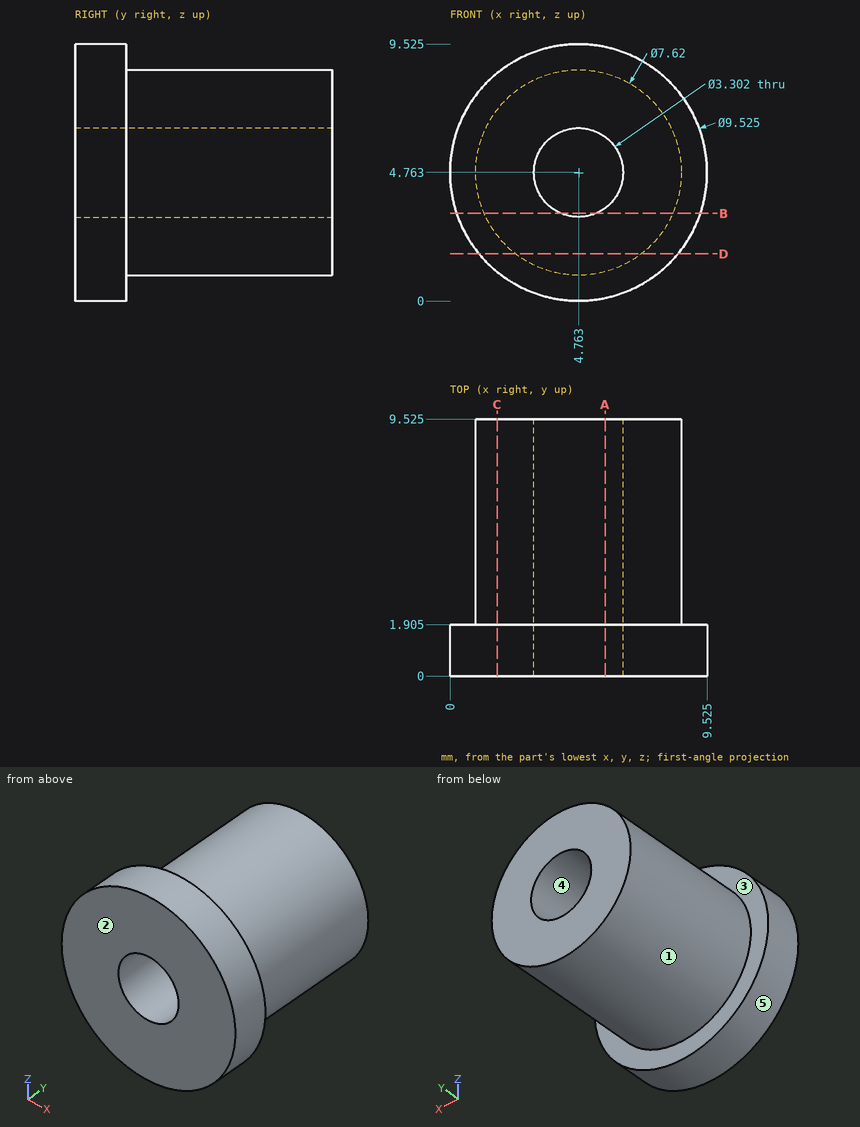
Geometry check sheet. Reference: drawing and pictorial views, mm from the part's lowest x, y, z. A direction names the side the tool comes from. Give positions to 0.01 mm unless a question says otherwise; leave off trailing zeros. Order: outer loops, then holes, each group sorted by start corner. A loop starts at its lowest first (then second) coordinate and runs counter-clockwise, first axis right, second up. Notation, with made-up numbers: M 8,31.5 L 54,31.5 A18 ccw 54,53.5 Z; hole C 40.25,58.5 d9. An arc over 180 degrees is marked long. Use one line per item in the form item = value. Start each with the question number.
Q1. Go/stop test with flat-tipped pins: pin 1 Ø1.5 at (y, z) = (5, 3) entering from -X; pin 2 Ø2 at (x, y) = (2.5, 1.5) entering from +Z (1 decimal); pin 3 Ø2 at (x, z) = (4.76, 4.76) entering from +Y; pin 4 Ø1.5 at (y, z) = (3.5, 7) entering from +X. Record where each tip stops, or that it passes through.
Q2. Scan lines: line 1 along X through (y, z) = (0.5, 4.75) (1 decimal); line 2 along X through (y, z) = (9, 4.75); line 3 along Z through (x, y) = (3.75, 5.5) (1 decimal). Record each from-to range of solid material in increasing order. Write a range as [from, to].
Q3. Section check C-C (x = 1.75). Enter the section's corners in (y, z) (1 decimal).
Q4. Mould release check, pull along Z, two halves, no side actions. Record for the marked faces 3, 4 and 5: +Z half, -Z half, draft (parallel to the pull), parting line (faces both ways), or undercut.
Q5. Access from +Z, -Z, +X, -X, +Y, -Y to the whole of each face (thin tool, end or side, straight path). Record for the marked faces 1 and 2.
Q6. Section check A-A (x = 5.75). Enter the section's corners in (y, z) (1 decimal).
Q7. Section check B-B (z = 3.25). Enter the section's corners in (x, y) (1 decimal).
Q8. Section check D-D (z = 1.75). Enter the section's corners in (x, y) (1 decimal), then the cut area to 3 significant figures.
Evaluation:
q1.pin_1 = 1.09
q1.pin_2 = 9.4
q1.pin_3 = through
q1.pin_4 = 8.27
q2.line_1 = [0, 3.1], [6.4, 9.5]
q2.line_2 = [0.95, 3.11], [6.41, 8.57]
q2.line_3 = [1.1, 3.5], [6.1, 8.4]
q3.outline = M 0,1.1 L 1.9,1.1 L 1.9,2.4 L 9.5,2.4 L 9.5,7.1 L 1.9,7.1 L 1.9,8.5 L 0,8.5 Z
q4.face_3 = draft
q4.face_4 = undercut
q4.face_5 = parting line
q5.face_1 = +Y
q5.face_2 = +Z, -Z, +X, -X, -Y
q6.outline = M 0,0.1 L 1.9,0.1 L 1.9,1.1 L 9.5,1.1 L 9.5,3.4 L 0,3.4 Z; M 0,6.1 L 9.5,6.1 L 9.5,8.4 L 1.9,8.4 L 1.9,9.4 L 0,9.4 Z
q7.outline = M 0.2,0 L 4.1,0 L 4.1,9.5 L 1.3,9.5 L 1.3,1.9 L 0.2,1.9 Z; M 5.4,0 L 9.3,0 L 9.3,1.9 L 8.3,1.9 L 8.3,9.5 L 5.4,9.5 Z
q8.outline = M 1.1,0 L 8.5,0 L 8.5,1.9 L 7.1,1.9 L 7.1,9.5 L 2.4,9.5 L 2.4,1.9 L 1.1,1.9 Z
q8.area = 49.6 mm2
